Design review of the part built by this model. Coordinates are the model's own, in mm. Coordinates: 2 decimals unless noted, no trailing zeros. Write each loop counter-clockwise with the first axis right and the second up, starting at its lowest first coordinate (ties: lowest second). Pieces come first, ordered by that corner, then holes.
Q1. For L1, parallel to Y at x = 176, z = 0.5; L2, parallel to X at y = -5, z = 3.9; L3, parallel to X at y = -1.5, z = 0.35, list the stretches that pass through material, from the lowest coordinate up.
Q2. Take a section at B-B, the plane x = 407.5. Write out the cut boundary in (y, z), plus the area to 3 significant figures.
Q3. Take a section at C-C, the plane y = 0. Write out the cut boundary in (x, z).
Q4. Take a section at A-A, the plane z = 2.5. Write out the cut boundary in (x, y).
Q5. For pin 1 Ø8 at (x, y) = (70, -19) entering from -Z; pin 2 Ø1 at (y, z) = (-16, 3) entering from +X; pin 3 Ø22.5 at (x, y) = (584.2, 0) entering from +Z, all flat-tipped, find the tip position at first contact; note any pin that passes through.
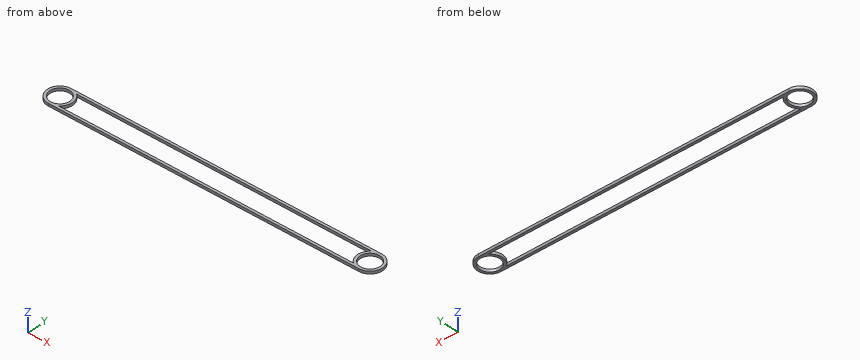
Autodesk Inventor part; units mm, degrees
ref_plane "YZ Plane" through (0, 0, 0) normal (1, 0, 0) x (0, 1, 0)
ref_plane "XZ Plane" through (0, 0, 0) normal (0, 1, 0) x (-1, 0, 0)
ref_plane "XY Plane" through (0, 0, 0) normal (0, 0, 1) x (1, 0, 0)
sketch "Sketch1" plane through (0, 0, 0) normal (0, 0, 1) x (1, 0, 0)
  circle A0 centre (0, 0) radius 18.8595
  arc A1 (0, 23.6903) -> (0, -23.6903) centre (0, 0) ccw
  circle A2 centre (584.2, 0) radius 18.8608
  arc A3 (569.8648, 18.8608) -> (569.8648, -18.8608) centre (584.2, 0) ccw
  line L0 (584.2, 23.6903) -> (0, 23.6903)
  line L1 (0, -23.6903) -> (584.2, -23.6903)
  line L2 (569.8648, -18.8608) -> (14.3352, -18.8608)
  line L3 (14.3352, 18.8608) -> (569.8648, 18.8608)
  arc A4 (14.3352, -18.8608) -> (14.3352, 18.8608) centre (0, 0) ccw
  arc A5 (584.2, -23.6903) -> (584.2, 23.6903) centre (584.2, 0) ccw
  dimension "d0" = 37.719
extrude "Extrusion1" add sketch "Sketch1" along normal blind 5.08
properties part number "false chain"
Responses:
1. L1: y = -23.69 to -18.86, 18.86 to 23.69
1. L2: x = -23.16 to -18.18, 18.18 to 23.16, 561.04 to 566.01, 602.39 to 607.36
1. L3: x = -23.64 to -18.8, 18.8 to 23.64, 560.56 to 565.4, 603 to 607.84
2. outline: (-23.69, 0) - (-18.86, 0) - (-18.86, 5.08) - (-23.69, 5.08) - close; (18.86, 0) - (23.69, 0) - (23.69, 5.08) - (18.86, 5.08) - close
2. area: 49.1 mm2
3. outline: (-23.69, 0) - (-18.86, 0) - (-18.86, 5.08) - (-23.69, 5.08) - close; (18.86, 0) - (23.69, 0) - (23.69, 5.08) - (18.86, 5.08) - close; (560.51, 0) - (565.34, 0) - (565.34, 5.08) - (560.51, 5.08) - close; (603.06, 0) - (607.89, 0) - (607.89, 5.08) - (603.06, 5.08) - close
4. outline: (0, -23.69) - (584.2, -23.69) arc R23.69 ccw to (584.2, 23.69) - (0, 23.69) arc R23.69 ccw to start; hole circle Ø37.72 at (0, 0); hole (14.34, -18.86) - (569.86, -18.86) arc R23.69 cw to (569.86, 18.86) - (14.34, 18.86) arc R23.69 cw to start; hole circle Ø37.72 at (584.2, 0)
5. pin 1: stops at z = 0
5. pin 2: stops at x = 602.12
5. pin 3: passes through
